```python
from build123d import *

# Parameters (mm, degrees)
F3_DEPTH = 73.8
F4_R     = 11
F5_DEPTH = 15


with BuildPart() as f1:
    # F0 (on Front) → F1 (revolve)
    with BuildSketch(Plane.XZ):
        Polygon((0, 10.5), (0, 0), (70, 0), (70, 12), (65.5, 16.5), (16.5, 16.5), (12, 12), (12, 10.5), align=None)
    revolve(axis=Axis((-7.5785342084, 0, 0), (-1, 0, 0)))

    # F2 (on face) → F3 (cut)
    with BuildSketch(Plane.YZ.offset(70)):
        with BuildLine():
            Line((-5.8094750193, -10.5), (-12.7279220614, -10.5))
            ThreePointArc((-12.7279220614, -10.5), (0, -16.5), (12.7279220614, -10.5))
            Line((12.7279220614, -10.5), (5.8094750193, -10.5))
            ThreePointArc((5.8094750193, -10.5), (0, -12), (-5.8094750193, -10.5))
        make_face()
        with BuildLine():
            Line((5.8094750193, -10.5), (-5.8094750193, -10.5))
            ThreePointArc((-5.8094750193, -10.5), (0, -12), (5.8094750193, -10.5))
        make_face()
    extrude(amount=-F3_DEPTH, mode=Mode.SUBTRACT)

    # F4 (on face) → F5 (cut)
    with BuildSketch(Plane(origin=(0, 0, -10.5), x_dir=(1, 0, 0), z_dir=(0, 0, -1))):
        with Locations((40, 0)):
            Circle(F4_R)
    extrude(amount=-F5_DEPTH, mode=Mode.SUBTRACT)


solid = f1.part
```
For this review, take the finished solid that the model builds, in its own axes (mm). A direction names the side the tool comes from. Coordinates: 2 decimals unless noted, no trailing zeros. Loops run counter-clockwise (first coordinate to the right, second up) from the corner with the lowest first, then second, coordinate; pieces in that order, holes last.
1. For line 1 (X direction, y = 0, z = -6.25); line 2 (X direction, y = -3, z = 10.75); line 3 (X direction, y = -8, z = -5.5), list the stretches that pass through material, from the lowest coordinate up.
2. Insertion check: P1, Ø5, axis at x = 57, y = -7.5, coming from the +Z side; P2, Ø4, axis at x = 41, y = -2, coming from the -Z side; P3, Ø2, axis at x = 60.5, z = -7.5, coming from the +Y side. Each pin has a flat end and moves straight along its axis. Give the tip position at first contact, or say it passes through.
3. Add section A-A, the plane z = 0. Give the boundary of the cut face in (x, y), then the cut area to 3 significant figures.
4. Add section C-C, the plane x = 25. Give the boundary of the cut face in (y, z).
5. For faces 4 (the flat face through (12, 0, 11)), 5 (the flat face through (0, 0, 0)), 6 (the cylindrical face through (50.161, 4.213, -3.105)), list the 3-axis set-ups (+Z, -Z, +X, -X, +Y, -Y) from which the entire face can be reached by the end or side of a thin tool; tool diameter is ignored.
6. Mouldability with a two-part tool opening along Y and no side actions: class faces 1 (the cylindrical face through (40.66, -0.52, 16.49)), 2 (the flat face through (40, 0, 4.5)), 3 (the flat face through (48, 9, -10.5)) as +Y half, -Y half, draft (parallel to the pull), parting line (faces both ways), or undercut.
7. Add section B-B, the plane x = 40. Give the boundary of the cut face in (y, z).
Result:
1. line 1: x = 0 to 29, 51 to 70
1. line 2: x = 12 to 70
1. line 3: x = 0 to 32.45, 47.55 to 70
2. P1: stops at z = 15.72
2. P2: stops at z = 4.5
2. P3: stops at y = 15.17
3. outline: (0, -10.5) - (12, -10.5) - (12, -12) - (16.5, -16.5) - (65.5, -16.5) - (70, -12) - (70, 12) - (65.5, 16.5) - (16.5, 16.5) - (12, 12) - (12, 10.5) - (0, 10.5) - close; hole circle Ø22 at (40, 0)
3. area: 1,750 mm2
4. outline: (-12.73, -10.5) - (12.73, -10.5) arc R16.5 ccw (long way) to start
5. face 4: -X
5. face 5: +Z, -Z, -X, +Y, -Y
5. face 6: -Z
6. face 1: parting line
6. face 2: undercut
6. face 3: draft
7. outline: (-12.73, -10.5) - (-11, -10.5) - (-11, 4.5) - (11, 4.5) - (11, -10.5) - (12.73, -10.5) arc R16.5 ccw (long way) to start
